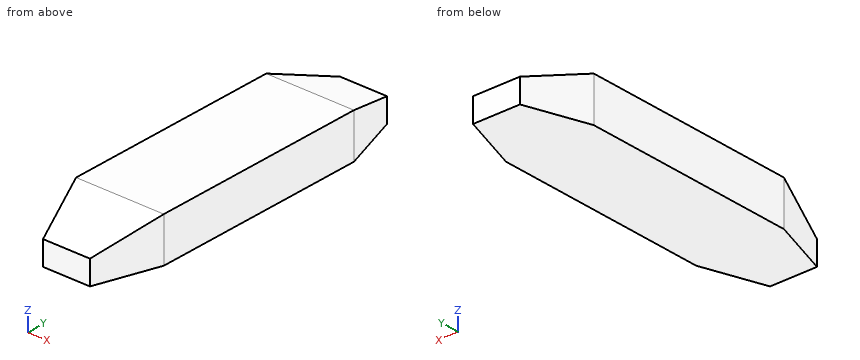
Autodesk Fusion 360 part; units mm, degrees
sketch "Sketch1" plane through (0, 0, 0) normal (0, 0, 1) x (1, 0, 0)
  line L0 (0, 0) -> (12.9, 0)
  line L1 (12.9, 0) -> (12.9, 50)
  line L2 (12.9, 50) -> (0, 50)
  line L3 (0, 50) -> (0, 0)
  dimension "d1" = 12.9
  dimension "d2" = 50
extrude "Extrude1" add sketch "Sketch1" along normal blind 6.5
chamfer "Chamfer1" distance 9 distance2 3 2 edges at (0, 0, 3.25) (12.9, 50, 3.25) measured on face at (0, 33.3333, 4.3333) measured on face at (12.9, 16.6667, 4.3333)
chamfer "Chamfer2" distance 3 distance2 9 2 edges at (12.9, 0, 3.25) (0, 50, 3.25) measured on face at (6.3, 0, 2.1667) measured on face at (6.6, 50, 2.1667)
chamfer "Chamfer3" distance 9 distance2 3 1 edges at (6.45, 50, 6.5) measured on face at (4.3, 19.6667, 6.5)
chamfer "Chamfer4" distance 9 distance2 3 1 edges at (6.45, 0, 6.5) measured on face at (4.3, 30.3333, 6.5)
equation "d5 = splinter"
equation "d8 = splinter"
equation "d9 = splinter"
equation "d11 = splinter"
equation "splinter = 9 mm"
Verification items for the finished model (mm, model axes). Round coordinates to 2 decimals unless told otherwise and drop trailing zeros. Order: outer loops, then holes, each group sorted by start corner. A loop starts at its lowest first (then second) coordinate and runs counter-clockwise, first axis right, second up. Notation, with made-up numbers: (-29, -2) -> (-8, -2) arc R9 ccw to (-8, 12) -> close; hole circle Ø1 at (56.5, 43). An arc over 180 degrees is marked (long way). Put each result on its own line as item: value. Start each with the question number.
(1) Section check A-A (z = 3). Enter the section's corners in (x, y), then the cut area to 3 significant figures.
(2) Section check D-D (z = 5). Enter the section's corners in (x, y), then the cut area to 3 significant figures.
(3) Section check C-C (y = 6). Enter the section's corners in (x, z), then the cut area to 4 significant figures.
(4) Section check B-B (x = 6). Enter the section's corners in (y, z), then the cut area to 3 significant figures.
(5) Material ranges on line 1 along Z through (x, y) = (3.5, 4); line 2 along X through (y, z) = (45.5, 1); line 3 along X through (y, z) = (6, 1), recorded low to high.
Completed:
1. outline: (0, 9) -> (3, 0) -> (9.9, 0) -> (12.9, 9) -> (12.9, 41) -> (9.9, 50) -> (3, 50) -> (0, 41) -> close
1. area: 591 mm2
2. outline: (0, 9) -> (1.5, 4.5) -> (11.4, 4.5) -> (12.9, 9) -> (12.9, 41) -> (11.4, 45.5) -> (1.5, 45.5) -> (0, 41) -> close
2. area: 515 mm2
3. outline: (1, 0) -> (11.9, 0) -> (11.9, 5.5) -> (1, 5.5) -> close
3. area: 59.95 mm2
4. outline: (0, 0) -> (50, 0) -> (50, 3.5) -> (41, 6.5) -> (9, 6.5) -> (0, 3.5) -> close
4. area: 298 mm2
5. line 1: z = 0 to 4.83
5. line 2: x = 1.5 to 11.4
5. line 3: x = 1 to 11.9
